from build123d import *

# Parameters (mm, degrees)
BOSS_EXTRUDE2_DEPTH = 45
BOSS_EXTRUDE3_DEPTH = 20
SKETCH3_W           = 5
SKETCH3_H           = 5
CUT_EXTRUDE1_DEPTH  = 25
SKETCH4_R           = 10
SKETCH4_R_2         = 5
CUT_EXTRUDE2_DEPTH  = 81.777472107


with BuildPart() as part:
    # Sketch1 → Boss-Extrude2 (new body)
    with BuildSketch(Plane(origin=(0, 0, 0), x_dir=(1, 0, 0), z_dir=(0, 1, 0))):
        with BuildLine():
            ThreePointArc((20, 0), (14.142135624, 14.142135624), (0, 20))
            ThreePointArc((0, 20), (-14.142135624, 14.142135624), (-20, 0))
            Line((-20, 0), (20, 0))
        make_face()
        with BuildLine():
            ThreePointArc((0, -20), (14.142135624, -14.142135624), (20, 0))
            Line((20, 0), (-20, 0))
            ThreePointArc((-20, 0), (-14.142135624, -14.142135624), (0, -20))
        make_face()
        with BuildLine():
            Line((20, -20), (20, -30))
            Line((20, -30), (60, -30))
            Line((60, -30), (60, 0))
            Line((60, 0), (20, 0))
            ThreePointArc((20, 0), (14.142135624, -14.142135624), (0, -20))
            Line((0, -20), (20, -20))
        make_face()
        with BuildLine():
            Line((60, 30), (20, 30))
            Line((20, 30), (20, 20))
            Line((20, 20), (0, 20))
            ThreePointArc((0, 20), (14.142135624, 14.142135624), (20, 0))
            Line((20, 0), (60, 0))
            Line((60, 0), (60, 30))
        make_face()
    extrude(amount=BOSS_EXTRUDE2_DEPTH)

    # Sketch1_3 → Boss-Extrude3 (add)
    with BuildSketch(Plane(origin=(0, 0, 0), x_dir=(1, 0, 0), z_dir=(0, 1, 0))):
        with BuildLine():
            Line((20, 30), (0, 30))
            ThreePointArc((0, 30), (-30, 0), (0, -30))
            Line((0, -30), (20, -30))
            Line((20, -30), (20, -20))
            Line((20, -20), (0, -20))
            ThreePointArc((0, -20), (-20, 0), (0, 20))
            Line((0, 20), (20, 20))
            Line((20, 20), (20, 30))
        make_face()
    extrude(amount=BOSS_EXTRUDE3_DEPTH)

    # Sketch3 → Cut-Extrude1 (cut)
    with BuildSketch(Plane(origin=(0, 45, 0), x_dir=(1, 0, 0), z_dir=(0, 1, 0))):
        with Locations((57.5, -27.5)):
            Rectangle(SKETCH3_W, SKETCH3_H)
        with Locations((57.5, 27.5)):
            Rectangle(SKETCH3_W, SKETCH3_H)
    extrude(amount=-CUT_EXTRUDE1_DEPTH, mode=Mode.SUBTRACT)

    # Sketch4 → Cut-Extrude2 (cut, through all)
    with BuildSketch(Plane(origin=(0, 45, 0), x_dir=(1, 0, 0), z_dir=(0, 1, 0))):
        with Locations(Location((0, 0, 0), (0, 0, 270))):
            Circle(SKETCH4_R)
        with Locations(Location((37.5, 15, 0), (0, 0, 270))):
            Circle(SKETCH4_R_2)
        with Locations(Location((37.5, -15, 0), (0, 0, 270))):
            Circle(SKETCH4_R_2)
    extrude(amount=-CUT_EXTRUDE2_DEPTH, mode=Mode.SUBTRACT)


solid = part.part
Design review of the part built by this model. Coordinates are the model's own, in mm. A direction names the side the tool comes from. Coordinates: 2 decimals unless noted, no trailing zeros. Loops run counter-clockwise (first coordinate to the right, second up) from the corner with the lowest first, then second, coordinate; pieces in that order, holes last. Notation, with made-up numbers: (52, 13.5) - (91, 13.5) arc R11 ccw to (91, 25.5) - close; hole circle Ø7 at (26, 46.25). An arc over 180 degrees is marked (long way). Use CSV: the item, a comma, the result in double quotes. Start each with the question number.
1. To check wall thickness, follow probe 1 along Z at (x, y) = (37, 11); probe 2 along X at (y, z) = (23, 0); probe 3 along Z at (x, y) = (36.5, 6.5). State the ranges of each line that lie inside material, in increasing order.
2. Add section A-A on x = 37.5. Give the boundary of the cut face in (y, z).
3. Add section D-D on x = -17. Give the boundary of the cut face in (y, z), plus the area to 3 significant figures.
4. For faces 5 (the flat face through (10, 32, -20)), 6 (the flat face through (57, 33, 25)), 7 (the flat face through (10, 32, 20)), list the 3-axis set-ups (+Z, -Z, +X, -X, +Y, -Y) from which the entire face can be reached by the end or side of a thin tool; tool diameter is ignored.
5. Clearance check with flat-ended pins moving along their axes: pin 1 (12 mm diameter, centred on y = 18.5, z = 23.5, fed in from -X); pin 2 (6 mm diameter, centred on x = 37.5, z = -15, fed in from +Y); pin 3 (5 mm diameter, centred on y = 33.5, z = 25.5, fed in from -X); pin 4 (2.5 mm diameter, centred on y = 35, z = -27.5, fed in from +X). State where each tip first meets the part, or that it passes through.
6. Add section C-C on y = 9.5. Give the boundary of the cut face in (x, z).
7. Add section B-B on z = 15. Give the boundary of the cut face in (x, y).
8. Mouldability with a two-part tool opening along Z and no side actions: class faces 1 (the cylindrical face through (-9.76, 22.82, -2.17)), 2 (the cylindrical face through (41.716, 22.815, 17.688)), 3 (the flat face through (28, 45, 0)), 4 (the cylindrical face through (-29.993, 9.86, -0.66)) as released by +Z, released by -Z, zero draft, split by the parting line, or undercut.
Resolved:
1,probe 1,"-30 to -19.97, -10.03 to 10.03, 19.97 to 30"
1,probe 2,"-20 to -10, 10 to 60"
1,probe 3,"-30 to -19.9, -10.1 to 10.1, 19.9 to 30"
2,outline,"(0, -30) - (45, -30) - (45, -20) - (0, -20) - close; (0, -10) - (45, -10) - (45, 10) - (0, 10) - close; (0, 20) - (45, 20) - (45, 30) - (0, 30) - close"
3,outline,"(0, -24.72) - (20, -24.72) - (20, -10.54) - (45, -10.54) - (45, 10.54) - (20, 10.54) - (20, 24.72) - (0, 24.72) - close"
3,area,"1,520 mm2"
4,face 5,"-Z, -X, +Y"
4,face 6,"+Z, +X, +Y"
4,face 7,"+Z, -X, +Y"
5,pin 1,"x = -24.37"
5,pin 2,"through"
5,pin 3,"x = 20"
5,pin 4,"x = 55"
6,outline,"(0, -30) - (60, -30) - (60, 30) - (0, 30) arc R30 ccw to start; hole circle Ø20 at (0, 0); hole circle Ø10 at (37.5, -15); hole circle Ø10 at (37.5, 15)"
7,outline,"(-25.98, 0) - (32.5, 0) - (32.5, 45) - (-13.23, 45) - (-13.23, 20) - (-25.98, 20) - close; (42.5, 0) - (60, 0) - (60, 45) - (42.5, 45) - close"
8,face 1,"undercut"
8,face 2,"undercut"
8,face 3,"zero draft"
8,face 4,"split by the parting line"
